Autodesk Inventor part; units mm, degrees
ref_plane "Work Plane1" through (0, 0, 52.5) normal (0, 0, -1) x (-1, 0, 0)
ref_plane "YZ Plane" through (0, 0, 0) normal (1, 0, 0) x (0, 1, 0)
ref_plane "XZ Plane" through (0, 0, 0) normal (0, 1, 0) x (-1, 0, 0)
sketch "Sketch1" plane through (0, 0, 0) normal (0, 0, 1) x (1, 0, 0)
  circle A0 centre (0, 0) radius 32.5
  dimension "d0" = 65
extrude "Extrusion1" add sketch "Sketch1" along normal blind 105
sketch "Sketch2" plane through (0, 0, 105) normal (0, 0, 1) x (1, 0, 0)
  circle A0 centre (0, 0) radius 27.5
  dimension "d3" = 55
extrude "Extrusion2" add sketch "Sketch2" along normal blind 20
sketch "Sketch3" plane through (0, 0, 125) normal (0, 0, 1) x (1, 0, 0)
  circle A0 centre (0, 0) radius 22.5
  dimension "d6" = 45
extrude "Extrusion3" add sketch "Sketch3" along normal blind 100
ref_plane "Work Plane1" through (0, 0, 52.5) normal (0, 0, -1) x (-1, 0, 0)
mirror "Mirror1" about plane through (0, 0, 52.5) normal (0, 0, -1) of "Extrusion3", "Extrusion2"
sketch "Sketch7" plane through (0, 0, -120) normal (0, 0, -1) x (-1, 0, 0)
  point P0 (0, 0)
sketch "Sketch11" plane through (0, 0, 52.5) normal (0, 0, -1) x (-1, 0, 0)
  circle A0 centre (0, 0) radius 35
  dimension "d43" = 70
extrude "Extrusion9" add sketch "Sketch11" along normal mid plane 65
sketch "Sketch12" plane through (0, 0, 225) normal (0, 0, 1) x (1, 0, 0)
  circle A0 centre (0, 0) radius 22.5
  line L0 (-19.6852, 6) -> (19.6852, 6)
  line L1 (21.6852, 4) -> (21.6852, -4)
  line L2 (19.6852, -6) -> (-19.6852, -6)
  line L3 (-21.6852, -4) -> (-21.6852, 4)
  arc A1 (-19.6852, 6) -> (-21.6852, 4) centre (-19.6852, 4) ccw
  arc A2 (-21.6852, -4) -> (-19.6852, -6) centre (-19.6852, -4) ccw
  arc A3 (19.6852, -6) -> (21.6852, -4) centre (19.6852, -4) ccw
  arc A4 (21.6852, 4) -> (19.6852, 6) centre (19.6852, 4) ccw
  point P0 (-21.6852, 6)
  point P1 (21.6852, 6)
  point P2 (21.6852, -6)
  point P3 (-21.6852, -6)
  dimension "d47" = 12
  dimension "d48" = 2
extrude "Extrusion10" add sketch "Sketch12" along normal blind 30 contours L0 A4 L1 A3 L2 A2 L3 A1
sketch "Sketch13" plane through (-19.6852, 6, 225) normal (0, 1, 0) x (1, 0, 0)
  circle A0 centre (19.6852, -15) radius 7.5
  line L0 (39.3705, -30) -> (0, -30)
  line L1 (39.3705, 0) -> (39.3705, -30)
  point P0 (19.6852, 225)
  dimension "d51" = 15
  dimension "d52" = 15
  dimension "d53" = 19.6852
extrude "Extrusion11" cut sketch "Sketch13" against normal through all
mirror "Mirror3" about plane through (0, 0, 52.5) normal (0, 0, -1) of "Extrusion10", "Extrusion11"
thread "Thread5"
sketch "Sketch14" plane through (0, 0, 225) normal (0, 0, 1) x (1, 0, 0)
  arc A0 (-21.6852, -4) -> (-19.6852, -6) centre (-19.6852, -4) ccw
  line L0 (-21.6852, -4) -> (-21.6852, 4)
  arc A1 (-19.6852, 6) -> (-21.6852, 4) centre (-19.6852, 4) ccw
  line L1 (-19.6852, 6) -> (19.6852, 6)
  arc A2 (21.6852, 4) -> (19.6852, 6) centre (19.6852, 4) ccw
  line L2 (21.6852, 4) -> (21.6852, -4)
  arc A3 (19.6852, -6) -> (21.6852, -4) centre (19.6852, -4) ccw
  line L3 (19.6852, -6) -> (-19.6852, -6)
  circle A4 centre (0, 0) radius 22.5
  line L4 (-19.6852, -6) -> (19.6852, -6)
  line L5 (-19.6852, -6) -> (-21.6852, -6)
  line L6 (19.6852, -6) -> (21.6852, -6)
extrude "Extrusion12" [suppressed]
sketch "Sketch15" plane through (0, 0, -120) normal (0, 0, -1) x (-1, 0, 0)
  arc A0 (19.6852, -6) -> (21.6852, -4) centre (19.6852, -4) ccw
  line L0 (19.6852, -6) -> (-19.6852, -6)
  arc A1 (-21.6852, -4) -> (-19.6852, -6) centre (-19.6852, -4) ccw
  line L1 (-21.6852, -4) -> (-21.6852, 4)
  arc A2 (-19.6852, 6) -> (-21.6852, 4) centre (-19.6852, 4) ccw
  line L2 (-19.6852, 6) -> (19.6852, 6)
  arc A3 (21.6852, 4) -> (19.6852, 6) centre (19.6852, 4) ccw
  line L3 (21.6852, 4) -> (21.6852, -4)
  circle A4 centre (0, 0) radius 22.5
  line L4 (-19.6852, -6) -> (-21.6852, -6)
  line L5 (19.6852, -6) -> (21.6852, -6)
extrude "Extrusion13" [suppressed]
sketch "Sketch16" plane through (0, 0, 255) normal (0, 0, 1) x (1, 0, 0)
  line L0 (-19.6852, -6) -> (19.6852, -6)
  arc A0 (19.6852, -6) -> (21.6852, -4) centre (19.6852, -4) ccw
  line L1 (21.6852, -4) -> (21.6852, 4)
  arc A1 (21.6852, 4) -> (19.6852, 6) centre (19.6852, 4) ccw
  line L2 (19.6852, 6) -> (-19.6852, 6)
  arc A2 (-19.6852, 6) -> (-21.6852, 4) centre (-19.6852, 4) ccw
  line L3 (-21.6852, 4) -> (-21.6852, -4)
  arc A3 (-21.6852, -4) -> (-19.6852, -6) centre (-19.6852, -4) ccw
  point P0 (0, 0)
extrude "Extrusion14" add sketch "Sketch16" along normal blind 10
sketch "Sketch17" plane through (19.6852, -6, -150) normal (0, 0, -1) x (-1, 0, 0)
  line L0 (39.3705, 0) -> (0, 0)
  arc A0 (39.3705, 0) -> (41.3705, 2) centre (39.3705, 2) ccw
  line L1 (41.3705, 10) -> (41.3705, 2)
  arc A1 (41.3705, 10) -> (39.3705, 12) centre (39.3705, 10) ccw
  line L2 (0, 12) -> (39.3705, 12)
  arc A2 (0, 12) -> (-2, 10) centre (0, 10) ccw
  line L3 (-2, 2) -> (-2, 10)
  arc A3 (-2, 2) -> (0, 0) centre (0, 2) ccw
  point P0 (19.6852, 6)
extrude "Extrusion15" add sketch "Sketch17" along normal blind 10
sketch "Sketch18" plane through (0, 0, 225) normal (0, 0, 1) x (1, 0, 0)
  arc A0 (-21.6852, -4) -> (-19.6852, -6) centre (-19.6852, -4) ccw
  line L0 (-21.6852, -4) -> (-21.6852, 4)
  arc A1 (-19.6852, 6) -> (-21.6852, 4) centre (-19.6852, 4) ccw
  line L1 (-19.6852, 6) -> (19.6852, 6)
  arc A2 (21.6852, 4) -> (19.6852, 6) centre (19.6852, 4) ccw
  line L2 (21.6852, 4) -> (21.6852, -4)
  arc A3 (19.6852, -6) -> (21.6852, -4) centre (19.6852, -4) ccw
  line L3 (19.6852, -6) -> (-19.6852, -6)
  circle A4 centre (0, 0) radius 22.5
  line L4 (-19.6852, 6) -> (-21.6852, 6)
  line L5 (19.6852, 6) -> (21.6852, 6)
extrude "Extrusion16" cut sketch "Sketch18" against normal blind 60 contours L4 A4 L5 L1
sketch "Sketch19" plane through (0, 0, -120) normal (0, 0, -1) x (-1, 0, 0)
  arc A0 (19.6852, -6) -> (21.6852, -4) centre (19.6852, -4) ccw
  line L0 (19.6852, -6) -> (-19.6852, -6)
  arc A1 (-21.6852, -4) -> (-19.6852, -6) centre (-19.6852, -4) ccw
  line L1 (-21.6852, -4) -> (-21.6852, 4)
  arc A2 (-19.6852, 6) -> (-21.6852, 4) centre (-19.6852, 4) ccw
  line L2 (-19.6852, 6) -> (19.6852, 6)
  arc A3 (21.6852, 4) -> (19.6852, 6) centre (19.6852, 4) ccw
  line L3 (21.6852, 4) -> (21.6852, -4)
  circle A4 centre (0, 0) radius 22.5
  line L4 (-19.6852, 6) -> (-21.6852, 6)
  line L5 (19.6852, 6) -> (21.6852, 6)
extrude "Extrusion17" cut sketch "Sketch19" against normal blind 60 contours L2 L4 A4 L5
properties part number "Shaft" material "Steel"
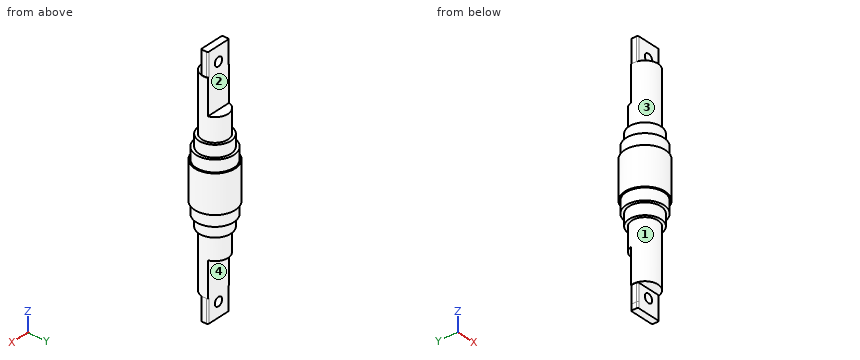
Design review of the part built by this model. Coordinates are the model's own, in mm. Face numbers are marked on the shaded views. A direction names the side the tool comes from. Give positions to 0.01 mm unless a question says otherwise; leave off trailing zeros. Order: outer loops, then holes, each group sorted by start corner. A loop starts at its lowest first (then second) coordinate and runs counter-clockwise, first axis right, second up. Notation, with made-up numbers: (-31, -19) - (-18, -19) arc R15 cw to (-18, -10) - close; hole circle Ø2 at (-20, 76). An arc over 180 degrees is marked (long way). Use CSV: the item, a comma, the result in double quotes. Start each with the question number.
Q1. For line 1 (Z direction, x = 0, y = 0); line 2 (Z direction, x = -1, y = 0); line 3 (X direction, y = -0.5, z = -135), list the stretches that pass through material, from the lowest coordinate up.
Q2. Take a section at B-B (x = 0). Count the separate pieces of the cut face and the enclosed holes in it, and give its area (3 significant figures).
Q3. Machinability: for the marked faces 1, 2, 3 and 4, which of the approach directions +Z, -Z, +X, -X, +Y, -Y give a long, thin tool a straight path to every point of the face, cutting with its end or side? Answer none if there is none.
Q4. For P1, Ø5, axis at x = -1, y = -19, coming from the +Z side; P2, Ø5, axis at x = 5, y = 14.5, coming from the -Z side; P3, Ø5, axis at x = 4.5, y = 14.5, coming from the +Z side, all flat-tipped, find the tip position at first contact; note any pin that passes through.
Q5. Take a section at C-C (y = 11). State the section outline as (x, z) points, and give its area (3 significant figures).
Q6. Take a section at A-A (z = -135). State the section outline as (x, y) points, and give its area (3 significant figures).
Q7. Take a section at D-D (z = 35). State the section outline as (x, y) points.
Calculated:
1,line 1,"z = -160 to -142.5, -127.5 to 232.5, 247.5 to 265"
1,line 2,"z = -160 to -142.43, -127.57 to 232.57, 247.43 to 265"
1,line 3,"x = -21.69 to -7.5, 7.5 to 21.69"
2,separate pieces,"3"
2,enclosed holes,"0"
2,area,"17,000 mm²"
3,face 1,"-Z"
3,face 2,"+Z, +X, -X, +Y"
3,face 3,"+Z"
3,face 4,"-Z, +X, -X, +Y"
4,P1,"stops at z = 225"
4,P2,"stops at z = -60"
4,P3,"stops at z = 165"
5,outline,"(-33.23, 20) - (-30.58, 20) - (-30.58, 0) - (-25.2, 0) - (-25.2, -20) - (-19.63, -20) - (-19.63, -60) - (19.63, -60) - (19.63, -20) - (25.2, -20) - (25.2, 0) - (30.58, 0) - (30.58, 20) - (33.23, 20) - (33.23, 85) - (30.58, 85) - (30.58, 105) - (25.2, 105) - (25.2, 125) - (19.63, 125) - (19.63, 165) - (-19.63, 165) - (-19.63, 125) - (-25.2, 125) - (-25.2, 105) - (-30.58, 105) - (-30.58, 85) - (-33.23, 85) - close"
5,area,"11,900 mm²"
6,outline,"(-21.69, -4) arc R2 ccw to (-19.69, -6) - (-7.5, -6) - (-7.5, 6) - (-19.69, 6) arc R2 ccw to (-21.69, 4) - close; (7.5, -6) - (19.69, -6) arc R2 ccw to (21.69, -4) - (21.69, 4) arc R2 ccw to (19.69, 6) - (7.5, 6) - close"
6,area,"337 mm²"
7,outline,"circle Ø70 at (0, 0)"
